Work out the finished part from the listing and answer in its coordinate system (mm). Give positions to 0.01 mm unless a question says otherwise; leave off trailing zeros. Write each loop counter-clockwise with the first axis right and the second up, starting at its lowest first coordinate (ties: lowest second). Pieces come first, ordered by that corner, then holes.
1) Straight lines are drawn through the part: probe 1 along Z at (x, y) = (1.5, 1.15); probe 2 along Z at (x, y) = (-21, 2.6); probe 3 along X at (y, z) = (2.6, 24). For each, find the intervals that lie inside material, in ascending order.
2) Given pin 1 Ø1.9 at (x, y) = (-49, 1) entering from -Z; pin 2 Ø1.4 at (y, z) = (1, 98) entering from +X; pin 3 Ø0.5 at (y, z) = (1.5, -98) entering from -X, each flat-ended and moving along its own axis, determine where each tip first touches the part or whether it passes through.
3) Find section D-D (z = 82.5). Determine the outline of the cut face in (x, y) (3 decimals), plus the area to 3 significant figures.
4) Find section B-B (z = -70.5). Determine the outline of the cut face in (x, y) (3 decimals), plus the area to 3 significant figures.
5) Find section C-C (x = 11). Determine the outline of the cut face in (y, z) (1 decimal), plus the area to 3 significant figures.
6) Find section A-A (x = 0). Determine the outline of the cut face in (y, z) (1 decimal).
```python
from build123d import *

# Parameters (mm, degrees)
SKETCH1_W                 = 100
SKETCH1_H                 = 198.069
BOSS_EXTRUDE1_DEPTH       = 3.175
SKETCH2_W                 = 14.285714286
SKETCH2_H                 = 3.18
ENDSLOTS_DEPTH            = 111.986092891
GIVEUPCORNER_DEPTH        = 111.986092891
GIVEUPCORNER_DEPTH_BACK   = 111.986092891
SKETCH6_W                 = 3.18
SKETCH6_H                 = 194.889
SKETCH3_W                 = 3.18
SKETCH3_H                 = 30
BOSS_EXTRUDE2_DEPTH       = 3.175
SKETCH4_W                 = 3.18
SKETCH4_H                 = 30
CUT_EXTRUDE2_DEPTH        = 111.986092891
SKETCH7_R                 = 1
CUT_EXTRUDE5_DEPTH        = 111.986092891
SKETCH_PATTERN1_DEPTH     = 3.175
CUT_EXTRUDE6_DEPTH        = 111.986092891
CUT_EXTRUDE6_DEPTH_BACK   = 111.986092891
SKETCH9_R                 = 1
SKETCH10_R                = 25
WEIGHTCUTOUT_DEPTH        = 111.986092891
ZSYMMETRY_COPY_1_SKETCH_R = 1
ZSYMMETRY_COPY_1_DEPTH    = 111.986092891
ZSYMMETRY_COPY_2_DEPTH    = 3.175
ZIPTIESLOTS_DEPTH         = 111.986092891
ZIPTIESLOTS_DEPTH_BACK    = 111.986092891
SKETCH5_W                 = 9.525
SKETCH5_H                 = 15
SKETCH5_W_2               = 12.705
FILLET1_R                 = 2


# Read off the part's stored shape, not the designer's step: Sketch-Pattern1
with BuildPart() as part:
    # Sketch1 → Boss-Extrude1 (new body)
    with BuildSketch(Plane(origin=(0, 0, 0), x_dir=(1, 0, 0), z_dir=(0, 1, 0))):
        Rectangle(SKETCH1_W, SKETCH1_H)
    extrude(amount=BOSS_EXTRUDE1_DEPTH)

    # Sketch2 → endSlots (cut, symmetric)
    with BuildSketch(Plane(origin=(0, 3.175, 0), x_dir=(1, 0, 0), z_dir=(0, 1, 0))):
        with Locations((-42.857142857, 97.4445)):
            Rectangle(SKETCH2_W, SKETCH2_H)
        with Locations((-14.285714286, 97.4445)):
            Rectangle(SKETCH2_W, SKETCH2_H)
        with Locations((14.285714286, 97.4445)):
            Rectangle(SKETCH2_W, SKETCH2_H)
        with Locations((42.857142857, 97.4445)):
            Rectangle(SKETCH2_W, SKETCH2_H)
    endslots = extrude(amount=ENDSLOTS_DEPTH, both=True, mode=Mode.SUBTRACT)

    # Sketch6 → giveUpCorner (cut, two sides: drawn at the far end of the back side and taken through both)
    with BuildSketch(Plane(origin=(0, 3.175, 0), x_dir=(1, 0, 0), z_dir=(0, 1, 0)).offset(-GIVEUPCORNER_DEPTH_BACK)):
        with Locations((48.41, -1.59)):
            Rectangle(SKETCH6_W, SKETCH6_H)
    extrude(amount=GIVEUPCORNER_DEPTH + GIVEUPCORNER_DEPTH_BACK, mode=Mode.SUBTRACT)

    # Sketch3 → Boss-Extrude2 (add)
    with BuildSketch(Plane(origin=(0, 3.175, 0), x_dir=(1, 0, 0), z_dir=(0, 1, 0))):
        with Locations((48.41, 47.13225)):
            Rectangle(SKETCH3_W, SKETCH3_H)
    boss_extrude2 = extrude(amount=-BOSS_EXTRUDE2_DEPTH)

    # Sketch4 → Cut-Extrude2 (cut, symmetric)
    with BuildSketch(Plane(origin=(0, 3.175, 0), x_dir=(1, 0, 0), z_dir=(0, 1, 0))):
        with Locations((-48.41, 47.13225)):
            Rectangle(SKETCH4_W, SKETCH4_H)
    cut_extrude2 = extrude(amount=CUT_EXTRUDE2_DEPTH, both=True, mode=Mode.SUBTRACT)

    # Sketch7 → Cut-Extrude5 (cut, symmetric)
    with BuildSketch(Plane(origin=(0, 3.175, 0), x_dir=(1, 0, 0), z_dir=(0, 1, 0))):
        with Locations((-36.421392495, 96.561606781)):
            Circle(SKETCH7_R)
    cut_extrude5 = extrude(amount=CUT_EXTRUDE5_DEPTH, both=True, mode=Mode.SUBTRACT)

    # Sketch-Pattern1 outline → Sketch-Pattern1 (cut)
    with BuildSketch(Plane(origin=(0, 0, 0), x_dir=(1, 0, 0), z_dir=(0, 1, 0))):
        with BuildLine():
            Line((-7.142857143, 95.8545), (-8.557070705, 95.8545))
            ThreePointArc((-8.557070705, 95.8545), (-7.849963924, 95.561606781), (-7.142857143, 95.8545))
        make_face()
        with BuildLine():
            Line((-7.142857143, 97.268713562), (-7.142857143, 95.8545))
            ThreePointArc((-7.142857143, 95.8545), (-6.849963924, 96.561606781), (-7.142857143, 97.268713562))
        make_face()
        with BuildLine():
            Line((21.428571429, 95.8545), (20.014357866, 95.8545))
            ThreePointArc((20.014357866, 95.8545), (20.721464647, 95.561606781), (21.428571429, 95.8545))
        make_face()
        with BuildLine():
            Line((21.428571429, 97.268713562), (21.428571429, 95.8545))
            ThreePointArc((21.428571429, 95.8545), (21.721464648, 96.561606781), (21.428571429, 97.268713562))
        make_face()
    sketch_pattern1 = extrude(amount=SKETCH_PATTERN1_DEPTH, mode=Mode.SUBTRACT)

    # Mirror3: Cut-Extrude5, Sketch-Pattern1 across plane
    add(cut_extrude5.mirror(Plane(origin=(0, 0, 0), x_dir=(0, 0, 1), z_dir=(1, 0, 0))), mode=Mode.SUBTRACT)
    add(sketch_pattern1.mirror(Plane(origin=(0, 0, 0), x_dir=(0, 0, 1), z_dir=(1, 0, 0))), mode=Mode.SUBTRACT)

    # Sketch9 → Cut-Extrude6 (cut, two sides: drawn at the far end of the back side and taken through both)
    with BuildSketch(Plane(origin=(0, 3.175, 0), x_dir=(1, 0, 0), z_dir=(0, 1, 0)).offset(-CUT_EXTRUDE6_DEPTH_BACK)):
        with Locations((-47.527106781, 61.425143219)):
            Circle(SKETCH9_R)
        with Locations((47.527106781, 31.425143219)):
            Circle(SKETCH9_R)
        with Locations((47.527106781, 62.839356781)):
            Circle(SKETCH9_R)
        with Locations((-47.527106781, 32.839356781)):
            Circle(SKETCH9_R)
    extrude(amount=CUT_EXTRUDE6_DEPTH + CUT_EXTRUDE6_DEPTH_BACK, mode=Mode.SUBTRACT)

    # Sketch10 → weightCutout (cut, symmetric)
    with BuildSketch(Plane(origin=(0, 3.175, 0), x_dir=(1, 0, 0), z_dir=(0, 1, 0))):
        with Locations(Location((0, 49.51725, 0), (0, 0, 270))):
            Circle(SKETCH10_R)
    weightcutout = extrude(amount=WEIGHTCUTOUT_DEPTH, both=True, mode=Mode.SUBTRACT)

    # zSymmetry: endSlots, Boss-Extrude2, Cut-Extrude2, Cut-Extrude5, Sketch-Pattern1, weightCutout across plane
    add(endslots.mirror(Plane.XY), mode=Mode.SUBTRACT)
    add(boss_extrude2.mirror(Plane.XY))
    add(cut_extrude2.mirror(Plane.XY), mode=Mode.SUBTRACT)
    add(cut_extrude5.mirror(Plane.XY), mode=Mode.SUBTRACT)
    add(sketch_pattern1.mirror(Plane.XY), mode=Mode.SUBTRACT)
    add(weightcutout.mirror(Plane.XY), mode=Mode.SUBTRACT)

    # zSymmetry copy 1 sketch → zSymmetry copy 1 (cut, symmetric)
    with BuildSketch(Plane(origin=(0, 3.175, 0), x_dir=(-1, 0, 0), z_dir=(0, 1, 0))):
        with Locations((-36.421392495, 96.561606781)):
            Circle(ZSYMMETRY_COPY_1_SKETCH_R)
    extrude(amount=ZSYMMETRY_COPY_1_DEPTH, both=True, mode=Mode.SUBTRACT)

    # zSymmetry copy 2 sketch → zSymmetry copy 2 (cut)
    with BuildSketch(Plane(origin=(0, 0, 0), x_dir=(-1, 0, 0), z_dir=(0, 1, 0))):
        with BuildLine():
            Line((-7.142857143, 95.8545), (-8.557070705, 95.8545))
            ThreePointArc((-8.557070705, 95.8545), (-7.849963924, 95.561606781), (-7.142857143, 95.8545))
        make_face()
        with BuildLine():
            Line((-7.142857143, 97.268713562), (-7.142857143, 95.8545))
            ThreePointArc((-7.142857143, 95.8545), (-6.849963924, 96.561606781), (-7.142857143, 97.268713562))
        make_face()
        with BuildLine():
            Line((21.428571429, 95.8545), (20.014357866, 95.8545))
            ThreePointArc((20.014357866, 95.8545), (20.721464647, 95.561606781), (21.428571429, 95.8545))
        make_face()
        with BuildLine():
            Line((21.428571429, 97.268713562), (21.428571429, 95.8545))
            ThreePointArc((21.428571429, 95.8545), (21.721464648, 96.561606781), (21.428571429, 97.268713562))
        make_face()
    extrude(amount=ZSYMMETRY_COPY_2_DEPTH, mode=Mode.SUBTRACT)

    # Sketch5 → zipTieSlots (cut, two sides: drawn at the far end of the back side and taken through both)
    with BuildSketch(Plane(origin=(0, 3.175, 0), x_dir=(1, 0, 0), z_dir=(0, 1, 0)).offset(-ZIPTIESLOTS_DEPTH_BACK)):
        with Locations((42.0575, 0)):
            Rectangle(SKETCH5_W, SKETCH5_H)
        with Locations((-43.6475, 0)):
            Rectangle(SKETCH5_W_2, SKETCH5_H)
    extrude(amount=ZIPTIESLOTS_DEPTH + ZIPTIESLOTS_DEPTH_BACK, mode=Mode.SUBTRACT)

    # Fillet1
    fillet1_edges = [part.edges().sort_by_distance(p)[0] for p in [
        (46.82, 1.5875, -7.5),
        (46.82, 1.5875, 7.5),
        (37.295, 1.5875, 7.5),
        (37.295, 1.5875, -7.5),
        (-50, 1.5875, 7.5),
        (-50, 1.5875, -7.5),
        (-37.295, 1.5875, -7.5),
        (-37.295, 1.5875, 7.5),
    ]]
    fillet(fillet1_edges, radius=FILLET1_R)


solid = part.part
```
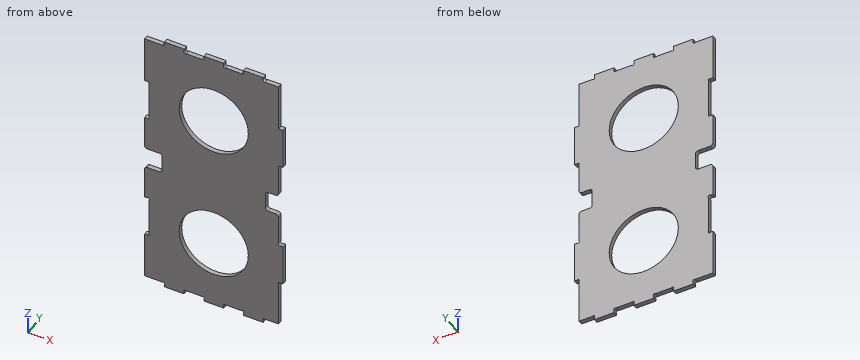
Results:
1. probe 1: z = -99.03 to -74.47, -24.56 to 24.56, 74.47 to 99.03
1. probe 2: z = -95.6 to -63.08, -35.95 to 35.95, 63.08 to 95.6
1. probe 3: x = -50 to 46.82
2. pin 1: stops at z = -95.85
2. pin 2: stops at x = 35.71
2. pin 3: stops at x = -35.71
3. outline: (-50, 0) - (46.82, 0) - (46.82, 3.175) - (-50, 3.175) - close
3. area: 307 mm2
4. outline: (-50, 0) - (-13.591, 0) - (-13.591, 3.175) - (-50, 3.175) - close; (13.591, 0) - (46.82, 0) - (46.82, 3.175) - (13.591, 3.175) - close
4. area: 221 mm2
5. outline: (0, -95.9) - (3.2, -95.9) - (3.2, -72) - (0, -72) - close; (0, -27.1) - (3.2, -27.1) - (3.2, 27.1) - (0, 27.1) - close; (0, 72) - (3.2, 72) - (3.2, 95.9) - (0, 95.9) - close
5. area: 324 mm2
6. outline: (0, -99) - (3.2, -99) - (3.2, -74.5) - (0, -74.5) - close; (0, -24.5) - (3.2, -24.5) - (3.2, 24.5) - (0, 24.5) - close; (0, 74.5) - (3.2, 74.5) - (3.2, 99) - (0, 99) - close
